Geometry check sheet. Reference: the model listing, model coordinates, mm. A direction names the side the tool comes from. Give positions to 0.01 mm unless a question says otherwise; leave off trailing zeros. Order: outer loops, then holes, each group sorted by start corner. A loop starts at its lowest first (then second) coordinate and runs counter-clockwise, first axis right, second up. Notation, with made-up numbers: M 47,56.25 L 101,56.25 A19 ccw 101,90.25 Z; hole C 73.25,0.25 d2. An arc over 180 degrees is marked long. Put each result on its own line as item: value. Start each with the question number.
Q1. Section check B-B on z = 5.9. Record the cut outline in (x, y), then the cut area to 3 significant figures.
Q2. Section check D-D on z = 20. Record the cut outline in (x, y), then the cut area to 3 significant figures.
Q3. Section check C-C on y = 13. State how many separate pieces and enclosed holes the cut face has, then the cut area to 3 significant figures.
Q4. Mould release check, pull along Z, two halves, no side actions. Record for faces 4 (the flat face through (0, 9, 30.9)), 5 (the flat face through (10, 12, 22)), 6 (the flat face through (6.942, 3, 6)): +Z half, -Z half, draft (parallel to the pull), parting line (faces both ways), or undercut.
Q5. Material ranges on L1, parallel to X at y = -1.65, z = 5.9; L2, parallel to Y at x = -17.5, z = -20.5; L3, parallel to Z at x = -12, y = 12.5, recorded low to high.
Q6. Section check A-A on x = -17.5. Record the cut outline in (y, z).
Q7. Access from +Z, -Z, +X, -X, +Y, -Y to the whole of each face (thin tool, end or side, straight path). Record for faces 1 (the flat face through (-25, 2, 0)), 2 (the flat face through (-10, 12, 22)), 3 (the flat face through (8.391, 3.028, 3.413)).
Q8. Go/stop test with flat-tipped pins: pin 1 (10 mm diameter, centred on x = 4.5, y = 17.5, fed in from -Z); pin 2 (5 mm diameter, centred on x = -3.5, z = -13, fed in from +Y); pin 3 (4.5 mm diameter, centred on x = -10, z = 5.5, fed in from +Y). Record where each tip stops, or that it passes through.
```python
from build123d import *

# Parameters (mm, degrees)
SKETCH1_W               = 50
SKETCH1_H               = 61.8
BOSS_EXTRUDE1_DEPTH     = 5
SKETCH2_W               = 15
SKETCH2_H               = 15
BOSS_EXTRUDE2_DEPTH     = 15
SKETCH3_R               = 5.05
CUT_EXTRUDE1_DEPTH      = 1
CUT_EXTRUDE1_DEPTH_BACK = 62.8
SKETCH4_W               = 20
SKETCH4_H               = 3
BOSS_EXTRUDE3_DEPTH     = 15
SKETCH6_W               = 50
SKETCH6_H               = 61.8
BOSS_EXTRUDE5_DEPTH     = 3
FILLET1_R               = 1
CUT_EXTRUDE2_DEPTH      = 4
M3_CLEARANCE_HOLE1_D    = 3.4


with BuildPart() as part:
    # Sketch1 → Boss-Extrude1 (new body)
    with BuildSketch(Plane(origin=(0, 0, 0), x_dir=(1, 0, 0), z_dir=(0, 1, 0))):
        Rectangle(SKETCH1_W, SKETCH1_H)
    extrude(amount=BOSS_EXTRUDE1_DEPTH)

    # Sketch2 → Boss-Extrude2 (add)
    with BuildSketch(Plane(origin=(0, 5, 0), x_dir=(1, 0, 0), z_dir=(0, 1, 0))):
        with Locations((-17.5, 23.4)):
            Rectangle(SKETCH2_W, SKETCH2_H)
        with Locations((17.5, 23.4)):
            Rectangle(SKETCH2_W, SKETCH2_H)
        with Locations((-17.5, -23.4)):
            Rectangle(SKETCH2_W, SKETCH2_H)
        with Locations((17.5, -23.4)):
            Rectangle(SKETCH2_W, SKETCH2_H)
    extrude(amount=BOSS_EXTRUDE2_DEPTH)

    # Sketch3 → Cut-Extrude1 (cut, two sides)
    with BuildSketch(Plane.XY.offset(30.9)) as cut_extrude1_sk:
        with Locations((-17.5, 13)):
            Circle(SKETCH3_R)
        with Locations((17.5, 13)):
            Circle(SKETCH3_R)
    extrude(amount=CUT_EXTRUDE1_DEPTH, mode=Mode.SUBTRACT)
    extrude(cut_extrude1_sk.sketch, amount=-CUT_EXTRUDE1_DEPTH_BACK, mode=Mode.SUBTRACT)

    # Sketch4 → Boss-Extrude3 (add)
    with BuildSketch(Plane(origin=(0, 5, 0), x_dir=(1, 0, 0), z_dir=(0, 1, 0))):
        with Locations((0, -29.4)):
            Rectangle(SKETCH4_W, SKETCH4_H)
    extrude(amount=BOSS_EXTRUDE3_DEPTH)

    # Sketch6 → Boss-Extrude5 (add)
    with BuildSketch(Plane.XZ):
        Rectangle(SKETCH6_W, SKETCH6_H)
    extrude(amount=BOSS_EXTRUDE5_DEPTH)

    # Fillet1
    fillet1_edges = [part.edges().sort_by_distance(p)[0] for p in [
        (-25, 5, 0),
        (-10, 5, -23.4),
        (-25, 20, -23.4),
        (-10, 20, -23.4),
        (10, 5, -23.4),
        (10, 20, -23.4),
        (-25, 20, 23.4),
        (25, 5, 0),
        (10, 5, 21.9),
        (25, 20, 23.4),
        (10, 20, 21.9),
        (-10, 20, 21.9),
        (-10, 5, 21.9),
        (-25, -3, 0),
        (25, -3, 0),
    ]]
    fillet(fillet1_edges, radius=FILLET1_R)

    # Sketch7 → Cut-Extrude2 (cut)
    with BuildSketch(Plane(origin=(0, 5, 0), x_dir=(1, 0, 0), z_dir=(0, 1, 0))):
        Polygon((-12.657883832, -4.25), (-12.657883832, -7.55), (-9.8, -9.2), (-6.942116168, -7.55), (-6.942116168, -4.25), (-9.8, -2.6), align=None)
        Polygon((12.657883832, -7.55), (12.657883832, -4.25), (9.8, -2.6), (6.942116168, -4.25), (6.942116168, -7.55), (9.8, -9.2), align=None)
    extrude(amount=-CUT_EXTRUDE2_DEPTH, mode=Mode.SUBTRACT)

    # M3 Clearance Hole1 (through all)
    with Locations(Plane(origin=(0, 5, 0), x_dir=(1, 0, 0), z_dir=(0, 1, 0))):
        with Locations((-9.8, -5.9), (9.8, -5.9)):
            Hole(M3_CLEARANCE_HOLE1_D / 2)


solid = part.part
```
Results found:
1. outline: M -25,-2 A1 ccw -24,-3 L -11.5,-3 L -11.5,1 L -12.66,1 L -12.66,5 L -24,5 A1 ccw -25,4 Z; M -8.1,-3 L 8.1,-3 L 8.1,1 L 6.94,1 L 6.94,5 L -6.94,5 L -6.94,1 L -8.1,1 Z; M 11.5,-3 L 24,-3 A1 ccw 25,-2 L 25,4 A1 ccw 24,5 L 12.66,5 L 12.66,1 L 11.5,1 Z
1. area: 326 mm^2
2. outline: M -25,-2 A1 ccw -24,-3 L 24,-3 A1 ccw 25,-2 L 25,19 A1 ccw 24,20 L 11,20 A1 ccw 10,19 L 10,6 A1 cw 9,5 L -9,5 A1 cw -10,6 L -10,19 A1 ccw -11,20 L -24,20 A1 ccw -25,19 Z; hole C -17.5,13 d10.1; hole C 17.5,13 d10.1
2. area: 689 mm^2
3. separate pieces: 7
3. enclosed holes: 0
3. area: 354 mm^2
4. face 4: +Z half
4. face 5: draft
4. face 6: undercut
5. L1: x = -25 to -11.5, -8.1 to 8.1, 11.5 to 25
5. L2: y = -3 to 7.95, 18.05 to 20
5. L3: z = -30.9 to -15.9, 15.9 to 30.9
6. outline: M -3,-30.9 L 7.95,-30.9 L 7.95,-15.9 L 5,-15.9 L 5,15.9 L 7.95,15.9 L 7.95,30.9 L -3,30.9 Z; M 18.05,-30.9 L 20,-30.9 L 20,-15.9 L 18.05,-15.9 Z; M 18.05,15.9 L 20,15.9 L 20,30.9 L 18.05,30.9 Z
7. face 1: +Z, -Z, -X, +Y, -Y
7. face 2: -Z, +Y
7. face 3: +Y
8. pin 1: stops at z = 27.9
8. pin 2: stops at y = 5
8. pin 3: stops at y = 1
